Geometry check sheet. Reference: the model listing, model coordinates, mm. A direction names the side the tool comes from. Round coordinates to 2 decimals unless told otherwise and drop trailing zeros. Order: outer loops, then holes, each group sorted by start corner. A loop starts at its lowest first (then second) coordinate and runs counter-clockwise, first axis right, second up. Notation, with made-up numbers: (84, 8.5) - (122, 8.5) arc R12 cw to (122, 24.5) - close; hole circle Ø8 at (44.25, 36.5). An arc over 180 degrees is marked (long way). Use a Markdown table: item, result. Add a question column.
(1) Section check B-B on y = 0. Record the boundary of the cut face in (x, z), then the cut area to 3 significant figures.
(2) Gauge pin test, flat ends, axial feed: P1, Ø3.5, axis at x = 14.35, y = 14.35, coming from the -Z side; P2, Ø19, axis at x = 6, y = 1.5, coming from the -Z side. Record the tip position at first contact, or that the pin passes through.
(3) Section check A-A on x = 26.25. Record the boundary of the cut face in (y, z).
(4) Thickness scan on line 1 along Y through (x, z) = (-26.25, 2.25); line 2 along X through (y, z) = (-18, 1). Record the ranges inside material, lowest first. Write a range as [from, to].
(5) Mould release check, pull along X, two halves, no side actions. Record for faces 3 (the face through (13, -10.75, 3)), 4 (the face through (-30.25, 0, 4)), 5 (the face through (0, -13, 8)), 6 (the face through (29.35, -29.39, 4.06)): released by +X, released by -X, zero draft, split by the parting line, or undercut.
(6) Access from +Z, -Z, +X, -X, +Y, -Y to the whole of each face (thin tool, end or side, straight path). Record for faces 1 (the face through (10.75, -9, 3)), 2 (the face through (-2, -20, 0)).
```python
from build123d import *

# Parameters (mm, degrees)
SKETCH_1_W          = 60.5
SKETCH_1_H          = 60.5
SKETCH_1_W_2        = 38.5
SKETCH_1_H_2        = 38.5
EXTRUDE_1_DEPTH     = 8
CUT_EXTRUDE_1_DEPTH = 2.35
SKETCH_3_R          = 1.6
CUT_EXTRUDE_2_DEPTH = 44.521546388
SKETCH_4_W          = 38.5
SKETCH_4_H          = 38.5
SKETCH_4_R          = 12.5
EXTRUDE_2_DEPTH     = 6.8
HOLE_WIZARD_M3_1_D  = 3.2
SKETCH_10_W         = 32
SKETCH_10_H         = 32
CUT_EXTRUDE_4_DEPTH = 0.5
SKETCH_11_W         = 4.5
SKETCH_11_H         = 8
SKETCH_11_W_2       = 5
SKETCH_11_H_2       = 3.75
CUT_EXTRUDE_6_DEPTH = 2
SKETCH_9_R          = 3
CUT_EXTRUDE_7_DEPTH = 5
FILLET_1_R          = 3


with BuildPart() as part:
    # ｽｹｯﾁ1 → ﾎﾞｽ - 押し出し1 (new body)
    with BuildSketch(Plane.XY):
        Rectangle(SKETCH_1_W, SKETCH_1_H)
        Rectangle(SKETCH_1_W_2, SKETCH_1_H_2, mode=Mode.SUBTRACT)
    extrude(amount=EXTRUDE_1_DEPTH)

    # ｽｹｯﾁ2 → ｶｯﾄ - 押し出し1 (cut)
    with BuildSketch(Plane(origin=(0, 0, 0), x_dir=(-1, 0, 0), z_dir=(0, 0, -1))):
        with BuildLine():
            Line((-19.25, 24.95), (19.25, 24.95))
            ThreePointArc((19.25, 24.95), (23.280508653, 23.280508653), (24.95, 19.25))
            Line((24.95, 19.25), (24.95, -19.25))
            ThreePointArc((24.95, -19.25), (23.280508653, -23.280508653), (19.25, -24.95))
            Line((19.25, -24.95), (-19.25, -24.95))
            ThreePointArc((-19.25, -24.95), (-23.280508653, -23.280508653), (-24.95, -19.25))
            Line((-24.95, -19.25), (-24.95, 19.25))
            ThreePointArc((-24.95, 19.25), (-23.280508653, 23.280508653), (-19.25, 24.95))
        make_face()
        with BuildLine():
            Line((-19.25, 20.75), (19.25, 20.75))
            ThreePointArc((19.25, 20.75), (20.310660172, 20.310660172), (20.75, 19.25))
            Line((20.75, 19.25), (20.75, -19.25))
            ThreePointArc((20.75, -19.25), (20.310660172, -20.310660172), (19.25, -20.75))
            Line((19.25, -20.75), (-19.25, -20.75))
            ThreePointArc((-19.25, -20.75), (-20.310660172, -20.310660172), (-20.75, -19.25))
            Line((-20.75, -19.25), (-20.75, 19.25))
            ThreePointArc((-20.75, 19.25), (-20.310660172, 20.310660172), (-19.25, 20.75))
        make_face(mode=Mode.SUBTRACT)
    extrude(amount=-CUT_EXTRUDE_1_DEPTH, mode=Mode.SUBTRACT)

    # ｽｹｯﾁ3 → ｶｯﾄ - 押し出し2 (cut, through all)
    with BuildSketch(Plane(origin=(0, 0, 0), x_dir=(-1, 0, 0), z_dir=(0, 0, -1))):
        with Locations((26.25, 26.25)):
            Circle(SKETCH_3_R)
        with Locations((26.25, -26.25)):
            Circle(SKETCH_3_R)
        with Locations((-26.25, -26.25)):
            Circle(SKETCH_3_R)
        with Locations((-26.25, 26.25)):
            Circle(SKETCH_3_R)
    extrude(amount=-CUT_EXTRUDE_2_DEPTH, mode=Mode.SUBTRACT)

    # ｽｹｯﾁ4 → ﾎﾞｽ - 押し出し2 (add)
    with BuildSketch(Plane.XY.offset(1.2)):
        Rectangle(SKETCH_4_W, SKETCH_4_H)
        Circle(SKETCH_4_R, mode=Mode.SUBTRACT)
    extrude(amount=EXTRUDE_2_DEPTH)

    # M3 すきま穴1 (through all)
    with Locations(Plane(origin=(0, 0, 1.2), x_dir=(-1, 0, 0), z_dir=(0, 0, -1))):
        with Locations((14.354267658, 14.354267658), (-14.354267658, 14.354267658), (-14.354267658, -14.354267658), (14.354267658, -14.354267658)):
            Hole(HOLE_WIZARD_M3_1_D / 2)

    # ｽｹｯﾁ10 → ｶｯﾄ - 押し出し4 (cut)
    with BuildSketch(Plane(origin=(0, 0, 1.2), x_dir=(-1, 0, 0), z_dir=(0, 0, -1))):
        Rectangle(SKETCH_10_W, SKETCH_10_H)
    extrude(amount=-CUT_EXTRUDE_4_DEPTH, mode=Mode.SUBTRACT)

    # ｽｹｯﾁ11 → ｶｯﾄ - 押し出し6 (cut)
    with BuildSketch(Plane(origin=(0, 0, 1.7), x_dir=(-1, 0, 0), z_dir=(0, 0, -1))):
        with Locations((13.5, 7.25)):
            Rectangle(SKETCH_11_W, SKETCH_11_H)
        with Locations((-13.25, -8.875)):
            Rectangle(SKETCH_11_W_2, SKETCH_11_H_2)
    extrude(amount=-CUT_EXTRUDE_6_DEPTH, mode=Mode.SUBTRACT)

    # ｽｹｯﾁ9 → ｶｯﾄ - 押し出し7 (cut)
    with BuildSketch(Plane(origin=(0, 0, 1.2), x_dir=(-1, 0, 0), z_dir=(0, 0, -1))):
        with Locations((14.354267658, 14.354267658)):
            Circle(SKETCH_9_R)
        with Locations((-14.354267658, 14.354267658)):
            Circle(SKETCH_9_R)
        with Locations((14.354267658, -14.354267658)):
            Circle(SKETCH_9_R)
        with Locations((-14.354267658, -14.354267658)):
            Circle(SKETCH_9_R)
    extrude(amount=-CUT_EXTRUDE_7_DEPTH, mode=Mode.SUBTRACT)

    # ﾌｨﾚｯﾄ1
    fillet_1_edges = [part.edges().sort_by_distance(p)[0] for p in [
        (30.25, -30.25, 4),
        (-30.25, -30.25, 4),
        (-30.25, 30.25, 4),
        (30.25, 30.25, 4),
    ]]
    fillet(fillet_1_edges, radius=FILLET_1_R)


solid = part.part
```
Check sheet entries:
| question | item | result |
|---|---|---|
| 1 | outline | (-30.25, 0) - (-24.95, 0) - (-24.95, 2.35) - (-20.75, 2.35) - (-20.75, 0) - (-19.25, 0) - (-19.25, 1.2) - (-16, 1.2) - (-16, 1.7) - (-12.5, 1.7) - (-12.5, 8) - (-30.25, 8) - close; (12.5, 1.7) - (16, 1.7) - (16, 1.2) - (19.25, 1.2) - (19.25, 0) - (20.75, 0) - (20.75, 2.35) - (24.95, 2.35) - (24.95, 0) - (30.25, 0) - (30.25, 8) - (12.5, 8) - close |
| 1 | area | 245 mm2 |
| 2 | P1 | stops at z = 6.2 |
| 2 | P2 | stops at z = 1.7 |
| 3 | outline | (-30.25, 0) - (-27.85, 0) - (-27.85, 8) - (-30.25, 8) - close; (-24.65, 0) - (24.65, 0) - (24.65, 8) - (-24.65, 8) - close; (27.85, 0) - (30.25, 0) - (30.25, 8) - (27.85, 8) - close |
| 4 | line 1 | y = [-30.25, -27.85], [-24.65, 24.65], [27.85, 30.25] |
| 4 | line 2 | x = [-30.25, -24.95], [-20.75, -19.25], [19.25, 20.75], [24.95, 30.25] |
| 5 | face 3 | undercut |
| 5 | face 4 | released by -X |
| 5 | face 5 | zero draft |
| 5 | face 6 | released by +X |
| 6 | face 1 | -Z |
| 6 | face 2 | -Z, +X, -X, +Y, -Y |
